```python
from build123d import *

# Parameters (mm, degrees)
F0_W     = 50.8
F0_H     = 30.48
F1_DEPTH = 50.8
F2_W     = 43.18
F2_H     = 21.59
F3_DEPTH = 45.72
F5_DEPTH = 5.08
F6_W     = 7.62
F6_H     = 45.72
F7_DEPTH = 13.47426
F8_W     = 30.48
F8_H     = 7.62
F9_DEPTH = 78.77304


with BuildPart() as f1:
    # F0 (on Top) → F1 (new body)
    with BuildSketch(Plane.XY):
        Rectangle(F0_W, F0_H)
    extrude(amount=F1_DEPTH)

    # F2 (on Top) → F3 (cut)
    with BuildSketch(Plane.XY):
        Rectangle(F2_W, F2_H)
    extrude(amount=F3_DEPTH, mode=Mode.SUBTRACT)

    # F4 (on face) → F5 (join)
    with BuildSketch(Plane.XY.offset(50.8)):
        Polygon((31.75, 15.24), (25.4, 15.24), (25.4, -15.24), (31.75, -15.24), (38.1, -15.24), (38.1, 15.24), align=None)
        with BuildLine():
            ThreePointArc((34.0614, -7.678979), (33.384407, -9.313385), (31.75, -9.990379))
            ThreePointArc((31.75, -9.990379), (30.115593, -6.044572), (34.0614, -7.678979))
        make_face(mode=Mode.SUBTRACT)
        with BuildLine():
            ThreePointArc((34.0614, 5.021021), (30.115593, 3.386615), (31.75, 7.332421))
            ThreePointArc((31.75, 7.332421), (33.384407, 6.655428), (34.0614, 5.021021))
        make_face(mode=Mode.SUBTRACT)
        with BuildLine():
            Line((-25.4, -15.24), (-25.4, 15.24))
            Line((-25.4, 15.24), (-31.75, 15.24))
            Line((-31.75, 15.24), (-38.1, 15.24))
            Line((-38.1, 15.24), (-38.1, -7.678979))
            Line((-38.1, -7.678979), (-34.0614, -7.678979))
            ThreePointArc((-34.0614, -7.678979), (-31.75, -5.367579), (-29.4386, -7.678979))
            ThreePointArc((-29.4386, -7.678979), (-30.115593, -9.313385), (-31.75, -9.990379))
            Line((-31.75, -9.990379), (-31.75, -15.24))
            Line((-31.75, -15.24), (-25.4, -15.24))
        make_face()
        with BuildLine():
            ThreePointArc((-29.4386, 5.021021), (-33.384407, 3.386615), (-31.75, 7.332421))
            ThreePointArc((-31.75, 7.332421), (-30.115593, 6.655428), (-29.4386, 5.021021))
        make_face(mode=Mode.SUBTRACT)
    extrude(amount=-F5_DEPTH)

    # F6 (on face) → F7 (cut)
    with BuildSketch(Plane(origin=(-25.4, 0, 0), x_dir=(0, -1, 0), z_dir=(-1, 0, 0))):
        with Locations((0, -22.86)):
            Rectangle(F6_W, F6_H)
        with Locations((0, 22.86)):
            Rectangle(F6_W, F6_H)
    extrude(amount=-F7_DEPTH, mode=Mode.SUBTRACT)

    # F8 (on face) → F9 (cut)
    with BuildSketch(Plane.YZ.offset(25.4)):
        with Locations((0, 3.81)):
            Rectangle(F8_W, F8_H)
        Polygon((26.814165, 7.62), (15.24, 7.62), (15.24, 0), (-15.24, 0), (-15.24, -4.411362), (26.814165, -4.411362), align=None)
    extrude(amount=-F9_DEPTH, mode=Mode.SUBTRACT)


solid = f1.part
```
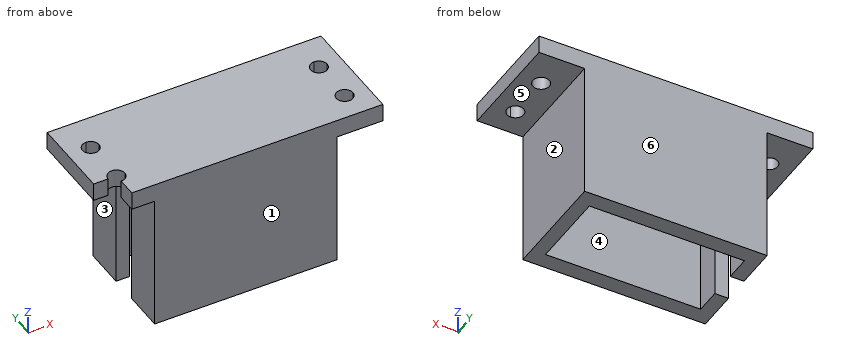
Could you check a few things on this model? Use its own coordinates, in mm. Face numbers are marked on the shaded views. A direction names the side the tool comes from. Round coordinates to 2 decimals unless told otherwise and drop trailing zeros. Write each loop counter-clockwise with the first axis right and the second up, starting at its lowest first coordinate (ties: lowest second). Pieces come first, ordered by that corner, then holes.
(1) Thinking about a two-plate mould opening in Y: for the marked faces 4, 5 and 6, which applies, +Y half, -Y half, draft (parallel to the pull), parting line (faces both ways), or undercut?
Findings below:
face 4: undercut
face 5: draft
face 6: +Y half
(2) Suppose I cut it at A-A on y = 1.5. Write out the boundary of the cut face in (x, z), and give its area (3 significant figures).
Findings below:
outline: (-38.1, 45.72) - (21.59, 45.72) - (21.59, 7.62) - (25.4, 7.62) - (25.4, 45.72) - (38.1, 45.72) - (38.1, 50.8) - (-38.1, 50.8) - close
area: 532 mm2
(3) For pin 1 (6 mm diameter, centred on y = 5, z = 25.5, fed in from +X); pin 2 (3 mm diameter, centred on x = -36, z = 48.5, fed in from -Y); pin 3 (9 mm diameter, centred on y = 9.5, z = 17, fed in from -X), each with a flat end and sliding along its axis, tell me the tip position at first contact or that it passes through.
Findings below:
pin 1: stops at x = 25.4
pin 2: stops at y = -7.68
pin 3: stops at x = -25.4
(4) Suppose I cut it at D-D on y = 10. Write out the boundary of the cut face in (x, z), and give its area (3 significant figures).
Findings below:
outline: (-38.1, 45.72) - (-25.4, 45.72) - (-25.4, 7.62) - (-21.59, 7.62) - (-21.59, 45.72) - (21.59, 45.72) - (21.59, 7.62) - (25.4, 7.62) - (25.4, 45.72) - (38.1, 45.72) - (38.1, 50.8) - (-38.1, 50.8) - close
area: 677 mm2
(5) Which directions (+Z, -Z, +X, -X, +Y, -Y) give clear straight access to the entire face, cutting with the end or side of a thin tool? Please do the marked faces 1, 2 and 3.
Findings below:
face 1: +Z, -Z, +X, -X, -Y
face 2: -Z, +X, +Y, -Y
face 3: -Z, -X, +Y, -Y
(6) Suppose I cut it at B-B on z = 43. Write out the boundary of the cut face in (x, y) (3 decimals), and give its area (3 significant figures).
Findings below:
outline: (-25.4, -15.24) - (25.4, -15.24) - (25.4, 15.24) - (-25.4, 15.24) - (-25.4, 3.81) - (-21.59, 3.81) - (-21.59, 10.795) - (21.59, 10.795) - (21.59, -10.795) - (-21.59, -10.795) - (-21.59, -3.81) - (-25.4, -3.81) - close
area: 587 mm2
(7) If I drill on probe 1 along Y at (x, z) = (2, 27) (3 decimals); probe 2 along X at (y, z) = (-4, 15.5); probe 3 along Y at (x, z) = (-31, 47), over which ranges is the centre line in solid material (lowest first)?
Findings below:
probe 1: y = -15.24 to -10.795, 10.795 to 15.24
probe 2: x = -25.4 to -21.59, 21.59 to 25.4
probe 3: y = -15.24 to -9.87, -5.49 to 2.83, 7.21 to 15.24
(8) Suppose I cut it at C-C on x = 13. Write out the boundary of the cut face in (y, z) (3 decimals), and give its area (3 significant figures).
Findings below:
outline: (-15.24, 7.62) - (-10.795, 7.62) - (-10.795, 45.72) - (10.795, 45.72) - (10.795, 7.62) - (15.24, 7.62) - (15.24, 50.8) - (-15.24, 50.8) - close
area: 494 mm2
